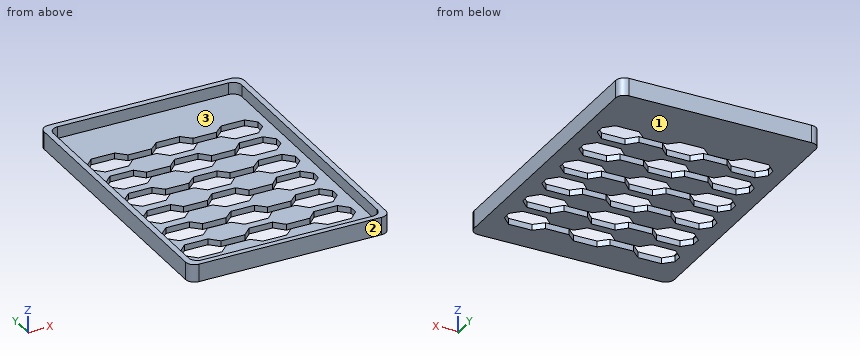
```python
from build123d import *

# Parameters (mm, degrees)
BOSS_EXTRUDE1_DEPTH = 6
BOSS_EXTRUDE2_DEPTH = 2


with BuildPart() as part:
    # Sketch1 → Boss-Extrude1 (new body)
    with BuildSketch(Plane(origin=(0, 0, 0), x_dir=(0, 1, 0), z_dir=(0, 0, 1))):
        with BuildLine():
            ThreePointArc((-45.5, -34), (-47.621320344, -33.121320344), (-48.5, -31))
            Line((-48.5, -31), (-48.5, 31))
            ThreePointArc((-48.5, 31), (-47.621320344, 33.121320344), (-45.5, 34))
            Line((-45.5, 34), (45.5, 34))
            ThreePointArc((45.5, 34), (47.621320344, 33.121320344), (48.5, 31))
            Line((48.5, 31), (48.5, -31))
            ThreePointArc((48.5, -31), (47.621320344, -33.121320344), (45.5, -34))
            Line((45.5, -34), (-45.5, -34))
        make_face()
        with BuildLine():
            Line((43.382784344, -32.008682641), (-43.617215656, -32.008682641))
            ThreePointArc((-43.617215656, -32.008682641), (-45.738535999, -31.130002985), (-46.617215656, -29.008682641))
            Line((-46.617215656, -29.008682641), (-46.617215656, 29.008682641))
            ThreePointArc((-46.617215656, 29.008682641), (-45.738535999, 31.130002985), (-43.617215656, 32.008682641))
            Line((-43.617215656, 32.008682641), (43.382784344, 32.008682641))
            ThreePointArc((43.382784344, 32.008682641), (45.504104688, 31.130002985), (46.382784344, 29.008682641))
            Line((46.382784344, 29.008682641), (46.382784344, -29.008682641))
            ThreePointArc((46.382784344, -29.008682641), (45.504104688, -31.130002985), (43.382784344, -32.008682641))
        make_face(mode=Mode.SUBTRACT)
    extrude(amount=BOSS_EXTRUDE1_DEPTH)

    # Sketch1_3 → Boss-Extrude2 (add)
    with BuildSketch(Plane(origin=(0, 0, 0), x_dir=(0, 1, 0), z_dir=(0, 0, 1))):
        with BuildLine():
            ThreePointArc((43.382784344, -32.008682641), (45.504104688, -31.130002985), (46.382784344, -29.008682641))
            Line((46.382784344, -29.008682641), (46.382784344, 29.008682641))
            ThreePointArc((46.382784344, 29.008682641), (45.504104688, 31.130002985), (43.382784344, 32.008682641))
            Line((43.382784344, 32.008682641), (-43.617215656, 32.008682641))
            ThreePointArc((-43.617215656, 32.008682641), (-45.738535999, 31.130002985), (-46.617215656, 29.008682641))
            Line((-46.617215656, 29.008682641), (-46.617215656, -29.008682641))
            ThreePointArc((-46.617215656, -29.008682641), (-45.738535999, -31.130002985), (-43.617215656, -32.008682641))
            Line((-43.617215656, -32.008682641), (43.382784344, -32.008682641))
        make_face()
        Polygon((-38.617215656, 18.008682641), (-38.617215656, 26.008682641), (-35.617215656, 29.008682641), (-32.617215656, 29.008682641), (-29.608533015, 26), (-29.608533015, 18), (-32.5, 15.108533015), (-32.5, 7), (-29.5, 4), (-29.5, -4), (-32.617231433, -6.999999928), (-32.564041089, -14.9998231), (-29.5, -18), (-29.5, -26), (-32.5, -29), (-35.5, -29), (-38.5, -26), (-38.5, -18), (-35.734431311, -15), (-35.734431311, -7), (-38.5, -4), (-38.5, 4), (-35.734431311, 7), (-35.734431311, 15), align=None, mode=Mode.SUBTRACT)
        Polygon((-17.734431311, -26), (-20.734431311, -29), (-23.734431311, -29), (-26.734431311, -26), (-26.734431311, -18), (-23.564091544, -14.998869032), (-23.617199878, -6.999999928), (-26.734431311, -4), (-26.734431311, 4), (-23.734431311, 7), (-23.734431311, 15.108533015), (-26.625898297, 18), (-26.625898297, 26), (-23.617215656, 29.008682641), (-20.617215656, 29.008682641), (-17.617215656, 26.008682641), (-17.617215656, 18.008682641), (-20.5, 15), (-20.5, 7), (-17.734431311, 4), (-17.734431311, -4), (-20.5, -7), (-20.5, -15), (-17.734431311, -18), align=None, mode=Mode.SUBTRACT)
        Polygon((-5.5, -4), (-8.617231433, -6.999999928), (-8.670339768, -14.998869032), (-5.5, -18), (-5.5, -26), (-8.5, -29), (-11.5, -29), (-14.5, -26), (-14.5, -18), (-11.734431311, -15), (-11.734431311, -7), (-14.5, -4), (-14.5, 4), (-11.734431311, 7), (-11.734431311, 15), (-14.617215656, 18.008682641), (-14.617215656, 26.008682641), (-11.617215656, 29.008682641), (-8.617215656, 29.008682641), (-5.608533015, 26), (-5.608533015, 18), (-8.5, 15.108533015), (-8.5, 7), (-5.5, 4), align=None, mode=Mode.SUBTRACT)
        Polygon((3.265568689, -29), (0.265568689, -29), (-2.734431311, -26), (-2.734431311, -18), (0.329609777, -14.9998231), (0.382800122, -6.999999928), (-2.734431311, -4), (-2.734431311, 4), (0.265568689, 7), (0.265568689, 15.108533015), (-2.625898297, 18), (-2.625898297, 26), (0.382784344, 29.008682641), (3.382784344, 29.008682641), (6.382784344, 26.008682641), (6.382784344, 18.008682641), (3.5, 15), (3.5, 7), (6.265568689, 4), (6.265568689, -4), (3.5, -7), (3.5, -15), (6.265568689, -18), (6.265568689, -26), align=None, mode=Mode.SUBTRACT)
        Polygon((15.5, -29), (12.5, -29), (9.5, -26), (9.5, -18), (12.265568689, -15), (12.265568689, -7), (9.5, -4), (9.5, 4), (12.265568689, 7), (12.265568689, 15), (9.382784344, 18.008682641), (9.382784344, 26.008682641), (12.382784344, 29.008682641), (15.382784344, 29.008682641), (18.391466985, 26), (18.391466985, 18), (15.5, 15.108533015), (15.5, 7), (18.5, 4), (18.5, -4), (15.382768567, -6.999999928), (15.435958911, -14.9998231), (18.5, -18), (18.5, -26), align=None, mode=Mode.SUBTRACT)
        Polygon((30.265568689, -26), (27.265568689, -29), (24.265568689, -29), (21.265568689, -26), (21.265568689, -18), (24.435908456, -14.998869032), (24.382800122, -6.999999928), (21.265568689, -4), (21.265568689, 4), (24.265568689, 7), (24.265568689, 15.108533015), (21.374101703, 18), (21.374101703, 26), (24.382784344, 29.008682641), (27.382784344, 29.008682641), (30.382784344, 26.008682641), (30.382784344, 18.008682641), (27.5, 15), (27.5, 7), (30.265568689, 4), (30.265568689, -4), (27.5, -7), (27.5, -15), (30.265568689, -18), align=None, mode=Mode.SUBTRACT)
    extrude(amount=BOSS_EXTRUDE2_DEPTH)


solid = part.part
```
Geometry check sheet. Reference: the model listing, model coordinates, mm. Face numbers are marked on the shaded views. Coordinates: 2 decimals unless noted, no trailing zeros. Order: outer loops, then holes, each group sorted by start corner. A loop starts at its lowest first (then second) coordinate and runs counter-clockwise, first axis right, second up.
Q1. Draft check along Y on the marked faces 1, 2 and 3. Enter one of: released by +Y, released by -Y, zero draft, split by the parting line, or undercut.
Reply:
face 1: zero draft
face 2: released by -Y
face 3: undercut
Q2. Sectioned sample at A-A on x = -24.5. Give the number of separate pieces and of enclosed holes in the cut face, and give its area (3 significant figures).
Reply:
separate pieces: 7
enclosed holes: 0
area: 102 mm2
Q3. Sectioned sample at D-D on y = 16.5. Record the cut outline in (x, z).
Reply:
outline: (-34, 0) - (-27.89, 0) - (-27.89, 2) - (-32.01, 2) - (-32.01, 6) - (-34, 6) - close; (-16.11, 0) - (-6, 0) - (-6, 2) - (-16.11, 2) - close; (5.92, 0) - (16.04, 0) - (16.04, 2) - (5.92, 2) - close; (28, 0) - (34, 0) - (34, 6) - (32.01, 6) - (32.01, 2) - (28, 2) - close
Q4. Sectioned sample at C-C on z = 3.75. Record the cut outline in (x, y), and give its area (3 significant figures).
Reply:
outline: (-34, -45.5) arc R3 ccw to (-31, -48.5) - (31, -48.5) arc R3 ccw to (34, -45.5) - (34, 45.5) arc R3 ccw to (31, 48.5) - (-31, 48.5) arc R3 ccw to (-34, 45.5) - close; hole (-32.01, -43.62) arc R3 ccw to (-29.01, -46.62) - (29.01, -46.62) arc R3 ccw to (32.01, -43.62) - (32.01, 43.38) arc R3 ccw to (29.01, 46.38) - (-29.01, 46.38) arc R3 ccw to (-32.01, 43.38) - close
area: 642 mm2
Q5. Thickness scan on probe 1 along X at (y, z) = (-11.5, 2.35); probe 2 along Y at (x, z) = (-12.5, 2.1); probe 3 along Z at (x, y) = (-14, -20). Record the ranges inside material, lowest first.
Reply:
probe 1: x = -34 to -32.01, 32.01 to 34
probe 2: y = -48.5 to -46.62, 46.38 to 48.5
probe 3: z = 0 to 2
Q6. Sectioned sample at B-B on y = -34.5. Record the cut outline in (x, z), and give its area (3 significant figures).
Reply:
outline: (-34, 0) - (-29.01, 0) - (-29.01, 2) - (-32.01, 2) - (-32.01, 6) - (-34, 6) - close; (29, 0) - (34, 0) - (34, 6) - (32.01, 6) - (32.01, 2) - (29, 2) - close
area: 35.9 mm2
Q7. Depth check by flat-ended pin: pin 1 Ø8 at (x, y) = (-23.5, -3) entering from +Z. Enter the tip coordinate at first touch or a pass-through.
Reply:
pin 1: stops at z = 2
